Could you check a few things on this model? Use its own coordinates, in mm. Round coordinates to 2 decimals unless told otherwise and drop trailing zeros. Loops run counter-clockwise (first coordinate to the right, second up) from the corner with the lowest first, then second, coordinate; pieces in that order, holes last. Notation, with made-up numbers: M 34.25,-8.75 L 63.25,-8.75 A36 cw 63.25,30.25 Z; hole C -35,76 d3. An arc over 180 degrees is marked long. Return JSON: item names as keys, results as strings. Group by question number.
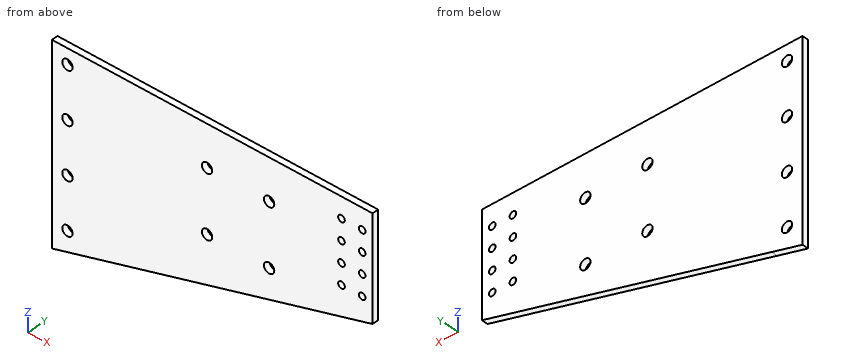
```python
from build123d import *

# Parameters (mm, degrees)
EXTRUDE_1_DEPTH             = 3
HOLE_WIZARD_5_0_5_2_D       = 5
HOLE_WIZARD_5_0_5_1_D       = 5
HOLE_WIZARD_3_2_3_2_2_D     = 3.2
PATTERN_LINEAR_1_COUNT      = 4
PATTERN_LINEAR_1_PITCH      = 10
PATTERN_LINEAR_1_COUNT_DIR2 = 2
PATTERN_LINEAR_1_PITCH_DIR2 = 10


with BuildPart() as part:
    # 草图1 → 凸台-拉伸1 (new body)
    with BuildSketch(Plane(origin=(0, 0, 0), x_dir=(1, 0, 0), z_dir=(0, 1, 0))):
        Polygon((-85, -45), (70, -45), (70, 5), (-70, 45), (-85, 45), align=None)
        Polygon((-85, 45), (-70, 45), (-85, 49.285714286), align=None)
    extrude(amount=EXTRUDE_1_DEPTH)

    # Ø5.0 (5) 直径孔2 (through all)
    with Locations(Plane(origin=(0, 3, 0), x_dir=(1, 0, 0), z_dir=(0, 1, 0))):
        with Locations((-77.5, -37.5), (-77.5, -12.5), (-77.5, 37.5), (-77.5, 12.5)):
            Hole(HOLE_WIZARD_5_0_5_2_D / 2)

    # Ø5.0 (5) 直径孔1 (through all)
    with Locations(Plane(origin=(0, 0, 0), x_dir=(-1, 0, 0), z_dir=(0, -1, 0))):
        with Locations((10, -25), (10, 5), (-20, 5), (-20, -25)):
            Hole(HOLE_WIZARD_5_0_5_1_D / 2)

    # Ø3.2 (3.2) 直径孔2 (through all)
    with Locations(Plane(origin=(0, 0, 0), x_dir=(-1, 0, 0), z_dir=(0, -1, 0))):
        with Locations((-65, -35)):
            hole_wizard_3_2_3_2_2 = Hole(HOLE_WIZARD_3_2_3_2_2_D / 2)

    # 阵列(线性)1: Hole Wizard 3.2 _3.2_ _2 4 × 2
    with Locations(*[(-j * PATTERN_LINEAR_1_PITCH_DIR2, 0, -i * PATTERN_LINEAR_1_PITCH) for i in range(PATTERN_LINEAR_1_COUNT) for j in range(PATTERN_LINEAR_1_COUNT_DIR2) if (i, j) != (0, 0)]):
        add(hole_wizard_3_2_3_2_2, mode=Mode.SUBTRACT)


solid = part.part
```
1. If we section it at B-B, the plane y = 2.05: Give the number of separate pieces and of enclosed holes in the cut face, then the cut area to 3 significant figures.
2. If we section it at A-A, the plane z = -12.5: Please give me the cut outline in (x, y).
3. I need wall thicknesses on probe 1 along Z at (x, y) = (18.5, 0.7); probe 2 along X at (y, z) = (1.8, 25); probe 3 along Z at (x, y) = (55, 2.4). Which ranges of each line are inside material? Lowest first, please.
4. If we section it at D-D, the plane x = 65: Please give me the cut outline in (y, z), then the cut area to 3 significant figures.
5. If we section it at C-C, the plane z = 25: Please give me the cut outline in (x, y), then the cut area to 3 significant figures.
Geometry results:
{
 "1": {"separate pieces": "1", "enclosed holes": "16", "area": "11,000 mm^2"},
 "2": {"outline": "M -85,0 L -80,0 L -80,3 L -85,3 Z; M -75,0 L 43.75,0 L 43.75,3 L -75,3 Z"},
 "3": {"probe 1": "-19.71 to -7, -3 to 23, 27 to 45", "probe 2": "-85 to -12.5, -7.5 to 17.5, 22.5 to 53.4, 56.6 to 63.4, 66.6 to 70", "probe 3": "-9.29 to 3.4, 6.6 to 13.4, 16.6 to 23.4, 26.6 to 33.4, 36.6 to 45"},
 "4": {"outline": "M 0,-6.43 L 3,-6.43 L 3,3.4 L 0,3.4 Z; M 0,6.6 L 3,6.6 L 3,13.4 L 0,13.4 Z; M 0,16.6 L 3,16.6 L 3,23.4 L 0,23.4 Z; M 0,26.6 L 3,26.6 L 3,33.4 L 0,33.4 Z; M 0,36.6 L 3,36.6 L 3,45 L 0,45 Z", "area": "116 mm^2"},
 "5": {"outline": "M -85,0 L -12.5,0 L -12.5,3 L -85,3 Z; M -7.5,0 L 17.5,0 L 17.5,3 L -7.5,3 Z; M 22.5,0 L 53.4,0 L 53.4,3 L 22.5,3 Z; M 56.6,0 L 63.4,0 L 63.4,3 L 56.6,3 Z; M 66.6,0 L 70,0 L 70,3 L 66.6,3 Z", "area": "416 mm^2"}
}
